Job drawing, mm, ordinate dimensions from the low corner. One solid piece. A direction names the side the tool comes from. Give positions to 0.01 mm unless a question says otherwise; leave off trailing zeros. Loops run counter-clockwise (first coordinate to the right, second up) from the corner with the lowest first, then second, coordinate; pieces in that order, holes last. Notation, with made-up numbers: (88.25, -17) -> (103.25, -17) arc R33 ccw to (103.25, 11) -> close; hole circle Ø1 at (9, -29.5). An arc over 180 degrees is marked (long way). Use one line per item in the form item = value.
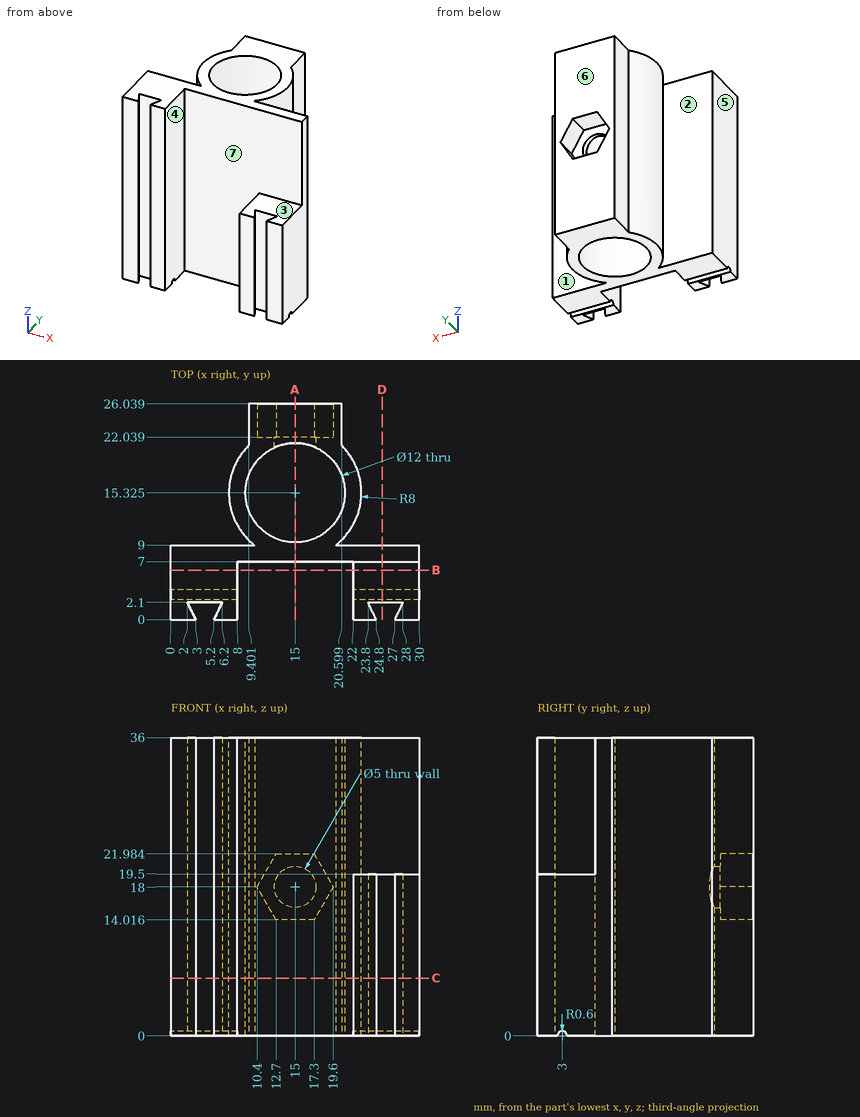
1. Cut at B-B, the plane y = 6. Write the cut outline in (x, z), then the cut area to 3 significant figures.
Result sheet:
outline = (0, 0) -> (8, 0) -> (8, 36) -> (0, 36) -> close; (22, 0) -> (30, 0) -> (30, 19.5) -> (22, 19.5) -> close
area = 444 mm^2
2. Drop flat-ended pins along their axis: P1, Ø5, axis at y = 13.5, z = 22, coming from the -X side; P2, Ø6, axis at x = 24, z = 24, coming from the +Y side (1 decimal); P3, Ø2, axis at y = 5, z = 30.5, coming from the +X side. Give the stop position or say it passes through.
Result sheet:
P1 = 7
P2 = 20.6
P3 = 8
3. Tool access for the marked faces 1, 2, 3 and 4: list every direction of +Z, -Z, +X, -X, +Y, -Y with a clear straight run to the whole face (end or side of a thin tool).
Result sheet:
face_1 = +Z, -Z, +X
face_2 = +Z, -Z, -X
face_3 = +Z, +X, -Y
face_4 = +Z, -Z, -Y
4. Mould opens along X. For the marked faces 5, 6 and 7 say: pulls with the +X half, pulls with the -X half, needs draft (parallel to the pull), parting line crosses it, or undercut.
Result sheet:
face_5 = pulls with the -X half
face_6 = needs draft
face_7 = undercut
5. Cut at A-A, the plane x = 15. Write the cut outline in (y, z) (1 decimal).
Result sheet:
outline = (7, 0) -> (9.3, 0) -> (9.3, 36) -> (7, 36) -> close; (21.3, 0) -> (26, 0) -> (26, 14) -> (22, 14) -> (22, 15.5) -> (21.3, 15.5) -> close; (21.3, 20.5) -> (22, 20.5) -> (22, 22) -> (26, 22) -> (26, 36) -> (21.3, 36) -> close
6. Cut at C-C, the plane z = 7. Write the cut outline in (x, y) (1 decimal).
Result sheet:
outline = (0, 0) -> (3, 0) -> (2, 2.1) -> (6.2, 2.1) -> (5.2, 0) -> (8, 0) -> (8, 7) -> (22, 7) -> (22, 0) -> (24.8, 0) -> (23.8, 2.1) -> (28, 2.1) -> (27, 0) -> (30, 0) -> (30, 9) -> (19.9, 9) arc R8 ccw to (20.6, 21) -> (20.6, 26) -> (9.4, 26) -> (9.4, 21) arc R8 ccw to (10.1, 9) -> (0, 9) -> close; hole circle Ø12 at (15, 15.3)
7. Cut at D-D, the plane x = 25.5. Write the cut outline in (y, z), then the cut area to 3 significant figures.
Result sheet:
outline = (2.1, 0) -> (2.4, 0) arc R0.6 cw to (3.6, 0) -> (9, 0) -> (9, 36) -> (7, 36) -> (7, 19.5) -> (2.1, 19.5) -> close
area = 167 mm^2
8. Drill centre lines: line 1 (X direction, y = 15, z = 31.5); line 2 (Y direction, x = 15, z = 24) (1 decimal); line 3 (Z direction, x = 15, y = 21.6). Where is each one in solid material? Low to high.
Result sheet:
line_1 = 7.01 to 9.01, 20.99 to 22.99
line_2 = 7 to 9.3, 21.3 to 26
line_3 = 0 to 15.5, 20.5 to 36
